from build123d import *

# Parameters (mm, degrees)
SKETCH_1_W          = 15
SKETCH_1_H          = 5
SKETCH_1_R          = 0.85
EXTRUDE_1_DEPTH     = 2
SKETCH_2_W          = 6
SKETCH_2_H          = 8
EXTRUDE_3_DEPTH     = 6
CUT_EXTRUDE_2_DEPTH = 8
SKETCH_7_W          = 5.1
SKETCH_7_H          = 5.1
CUT_EXTRUDE_3_DEPTH = 2
SKETCH_10_W         = 8
SKETCH_10_H         = 5.852977749
SKETCH_10_W_2       = 5.1
SKETCH_10_H_2       = 5.1
EXTRUDE_4_DEPTH     = 5
SKETCH_11_W         = 6
SKETCH_11_H         = 8
EXTRUDE_5_DEPTH     = 3
CUT_EXTRUDE_4_DEPTH = 5
SKETCH_13_W         = 4.5
SKETCH_13_H         = 5
CUT_EXTRUDE_5_DEPTH = 2


with BuildPart() as part:
    # 草图1 → 凸台-拉伸1 (new body)
    with BuildSketch(Plane(origin=(0, 0, 0), x_dir=(1, 0, 0), z_dir=(0, 1, 0))):
        with Locations((7.5, 2.5)):
            Rectangle(SKETCH_1_W, SKETCH_1_H)
        with Locations(Location((3.25, 2.5, 0), (0, 0, 270))):
            Circle(SKETCH_1_R, mode=Mode.SUBTRACT)
        with Locations(Location((11.75, 2.5, 0), (0, 0, 90))):
            Circle(SKETCH_1_R, mode=Mode.SUBTRACT)
    extrude(amount=EXTRUDE_1_DEPTH)

    # 草图2 → 凸台-拉伸3 (add)
    with BuildSketch(Plane.XZ):
        with Locations((7.5, -2.5)):
            Rectangle(SKETCH_2_W, SKETCH_2_H)
    extrude(amount=EXTRUDE_3_DEPTH)

    # 草图6 → 切除-拉伸2 (cut)
    with BuildSketch(Plane(origin=(0, 0, -6.5), x_dir=(-1, 0, 0), z_dir=(0, 0, -1))):
        Polygon((-10.5, -0.5), (-10.5, -6), (-8.498163712, -6), align=None)
    extrude(amount=-CUT_EXTRUDE_2_DEPTH, mode=Mode.SUBTRACT)

    # 草图7 → 切除-拉伸3 (cut)
    with BuildSketch(Plane(origin=(9.432430229, -3.43312384, 0), x_dir=(0, 0, -1), z_dir=(0.9396926207859104, -0.3420201433256631, 0))):
        with Locations((2.5, 0.19487632)):
            Rectangle(SKETCH_7_W, SKETCH_7_H)
    extrude(amount=-CUT_EXTRUDE_3_DEPTH, mode=Mode.SUBTRACT)

    # 草图10 → 凸台-拉伸4 (add)
    with BuildSketch(Plane(origin=(9.432430229, -3.43312384, 0), x_dir=(0, 0, -1), z_dir=(0.9396926207859104, -0.3420201433256631, 0))):
        with Locations((2.5, 0.19487632)):
            Rectangle(SKETCH_10_W, SKETCH_10_H)
        with Locations((2.5, 0.19487632)):
            Rectangle(SKETCH_10_W_2, SKETCH_10_H_2, mode=Mode.SUBTRACT)
    extrude(amount=EXTRUDE_4_DEPTH)

    # 草图11 → 凸台-拉伸5 (add)
    with BuildSketch(Plane(origin=(0, 0, 0), x_dir=(1, 0, 0), z_dir=(0, 1, 0))):
        with Locations((7.5, 2.5)):
            Rectangle(SKETCH_11_W, SKETCH_11_H)
    extrude(amount=EXTRUDE_5_DEPTH)

    # 草图12 → 切除-拉伸4 (cut)
    with BuildSketch(Plane(origin=(0, 3, 0), x_dir=(1, 0, 0), z_dir=(0, 1, 0))):
        with BuildLine():
            ThreePointArc((8.8, 2.5), (7.5, 3.8), (6.2, 2.5))
            Line((6.2, 2.5), (8.8, 2.5))
        make_face()
        with BuildLine():
            Line((8.8, 2.5), (6.2, 2.5))
            ThreePointArc((6.2, 2.5), (7.5, 1.2), (8.8, 2.5))
        make_face()
    extrude(amount=-CUT_EXTRUDE_4_DEPTH, mode=Mode.SUBTRACT)

    # 草图13 → 切除-拉伸5 (cut)
    with BuildSketch(Plane(origin=(0, 2, 0), x_dir=(1, 0, 0), z_dir=(0, 1, 0))):
        with Locations((2.25, 2.5)):
            Rectangle(SKETCH_13_W, SKETCH_13_H)
        with Locations((12.75, 2.5)):
            Rectangle(SKETCH_13_W, SKETCH_13_H)
    extrude(amount=-CUT_EXTRUDE_5_DEPTH, mode=Mode.SUBTRACT)


solid = part.part
Input: part model. Units: mm. Frame: model coordinates. A direction names the side the tool comes from. Give positions to 0.01 mm unless a question says otherwise; leave off trailing zeros. Write each loop counter-clockwise with the first axis right and the second up, starting at its lowest first coordinate (ties: lowest second). Pieces come first, ordered by that corner, then holes. Notation, with made-up numbers: M 9.25,16.25 L 32.25,16.25 A23 cw 32.25,36.25 Z; hole C 5,-38 d11. An arc over 180 degrees is marked long. Write item = value, one per line. Start each with the question number.
1) Material intervals for line 1 along X through (y, z) = (1.6, -2.5); line 2 along Z through (x, y) = (7.5, -0.35); line 3 along X through (y, z) = (2.25, -2), sorted ascending. Write a range as [from, to].
2) Cut plane D-D on x = 14. Return the cut outline in (y, z), then the cut area to 3 significant figures.
3) Draft query along Y for faces 1 (the flat face through (4.5, -2, -2)), 2 (the flat face through (7.44, -3.06, -2.46)), 3 (the flat face through (12.816, -1.343, -2.444)), 4 (the flat face through (6, -6, -2)). Return one class per face: +Y half, -Y half, draft (parallel to the pull), parting line (faces both ways), or undercut.
4) Reachability of faces 5 (the flat face through (11.73, -1.35, -2.46)), 6 (the flat face through (7, -2, -3)), 7 (the flat face through (9.99, -6.142, -2.464)) from +Z, -Z, +X, -X, +Y, -Y: full face, straight path, thin tool, end or side. Return the list, or none.
5) Cut plane C-C on z = -5.75. Return the cut outline in (x, y), then the cut area to 3 significant figures.
6) First-contact query: pin 1 Ø3 at (y, z) = (2, -4) entering from +X; pin 2 Ø3 at (x, z) = (6, -2.5) entering from -Y; pin 3 Ø0.8 at (x, z) = (7, -3) entering from +Y. Flat tips, straight axial feed; report the tip coordinate or a pass-through.
7) Cut plane B-B on x = 7.5. Return the cut outline in (y, z).
8) Cut plane A-A on z = -2.5. Return the cut outline in (x, y), then the cut area to 3 significant figures.
Solved:
q1.line_1 = [4.5, 6.2], [8.8, 10.5]
q1.line_2 = [-6.5, -3.8], [-1.2, 1.5]
q1.line_3 = [4.5, 6.3], [8.7, 10.5]
q2.outline = M -5.5,-6.5 L -1.77,-6.5 L -1.77,1.5 L -5.5,1.5 L -5.5,0.05 L -2.17,0.05 L -2.17,-5.05 L -5.5,-5.05 Z
q2.area = 12.9 mm2
q3.face_1 = draft
q3.face_2 = undercut
q3.face_3 = +Y half
q3.face_4 = -Y half
q4.face_5 = none
q4.face_6 = +Y
q4.face_7 = +X
q5.outline = M 4.5,-6 L 8.5,-6 L 13.2,-7.71 L 15.2,-2.21 L 10.5,-0.5 L 10.5,3 L 4.5,3 Z
q5.area = 77.8 mm2
q6.pin_1 = 10.5
q6.pin_2 = -6
q6.pin_3 = -2
q7.outline = M -6,-6.5 L 3,-6.5 L 3,-3.8 L -2,-3.8 L -2,-1.2 L 3,-1.2 L 3,1.5 L -6,1.5 Z; hole M -5.24,-5.05 L -2.89,-5.05 L -2.89,0.05 L -5.24,0.05 Z
q8.outline = M 4.5,-6 L 8.5,-6 L 13.2,-7.71 L 13.33,-7.36 L 6.75,-4.96 L 7.83,-2 L 6.2,-2 L 6.2,3 L 4.5,3 Z; M 8.8,-0.28 L 15.07,-2.56 L 15.2,-2.21 L 10.5,-0.5 L 10.5,3 L 8.8,3 Z
q8.area = 30.2 mm2
